Here's how the part is built. I have some questions about the finished solid (model axes, mm). A direction names the side the tool comes from. Coordinates: 2 decimals unless noted, no trailing zeros. Loops run counter-clockwise (first coordinate to the right, second up) from the corner with the lowest first, then second, coordinate; pieces in that order, holes last.
```python
from build123d import *

# Parameters (mm, degrees)
BOSS_EXTRUDE1_DEPTH = 12
CUT_EXTRUDE1_DEPTH  = 2
SKETCH3_W           = 16.6
SKETCH3_H           = 13.4
BOSS_EXTRUDE2_DEPTH = 5.2
SKETCH5_R           = 1.6
CUT_EXTRUDE2_DEPTH  = 5
SKETCH6_W           = 5
SKETCH6_H           = 4
BOSS_EXTRUDE4_DEPTH = 8
CUT_EXTRUDE4_DEPTH  = 7
SKETCH8_R           = 2.65
CUT_EXTRUDE5_DEPTH  = 7
SKETCH10_R          = 2.65
CUT_EXTRUDE6_DEPTH  = 7
CHAMFER2_SIZE       = 2
CHAMFER3_SIZE       = 1
SKETCH12_W          = 3
SKETCH12_H          = 2
SKETCH12_W_2        = 6.148694825
SKETCH12_W_3        = 1.851305175
BOSS_EXTRUDE5_DEPTH = 8
SKETCH13_R          = 2.65
CUT_EXTRUDE7_DEPTH  = 3
CHAMFER4_SIZE       = 5
CHAMFER4_SIZE_2     = 6.174485783
SKETCH16_W          = 1.5
SKETCH16_H          = 10
CUT_EXTRUDE8_DEPTH  = 11
CHAMFER5_SIZE       = 0.4


with BuildPart() as part:
    # Sketch1 → Boss-Extrude1 (new body)
    with BuildSketch(Plane(origin=(0, 0, 0), x_dir=(1, 0, 0), z_dir=(0, 1, 0))):
        with BuildLine():
            Line((-23.25, -5), (-5.749755012, -5))
            Line((-5.749755012, -5), (-5.749755012, 0))
            add(Edge.make_bspline(
                [(-3.25, 5), (-5.749755012, 5), (-5.749755012, 0)],
                knots=[0, 0, 0, 1.570796327, 1.570796327, 1.570796327], degree=2, weights=[1, 0.707106781, 1]))
            Line((-3.25, 5), (3.25, 5))
            add(Edge.make_bspline(
                [(5.748694825, 0), (5.748694825, 5), (3.25, 5)],
                knots=[4.71238898, 4.71238898, 4.71238898, 6.283185307, 6.283185307, 6.283185307], degree=2, weights=[1, 0.707106781, 1]))
            Line((5.748694825, 0), (5.748694825, -5))
            Line((5.748694825, -5), (23.25, -5))
            Line((23.25, -5), (23.25, -3))
            Line((23.25, -3), (23.25, -1))
            Line((23.25, -1), (9.3, -1))
            ThreePointArc((9.3, -1), (8.592893219, -0.707106781), (8.3, 0))
            Line((8.3, 0), (8.3, 6.6))
            Line((8.3, 6.6), (-8.3, 6.6))
            Line((-8.3, 6.6), (-8.3, 0))
            ThreePointArc((-8.3, 0), (-8.592893219, -0.707106781), (-9.3, -1))
            Line((-9.3, -1), (-23.25, -1))
            Line((-23.25, -1), (-23.25, -5))
        make_face()
    extrude(amount=BOSS_EXTRUDE1_DEPTH)

    # Sketch2 → Cut-Extrude1 (cut)
    with BuildSketch(Plane(origin=(0, 0, 1), x_dir=(-1, 0, 0), z_dir=(0, 0, -1))):
        Polygon((20.147177825, 6), (18.213054423, 9.35), (14.344807619, 9.35), (12.410684218, 6), (14.344807619, 2.65), (18.213054423, 2.65), align=None)
        Polygon((-12.542169585, 6), (-14.476292987, 9.35), (-18.34453979, 9.35), (-20.278663192, 6), (-18.34453979, 2.65), (-14.476292987, 2.65), align=None)
    extrude(amount=-CUT_EXTRUDE1_DEPTH, mode=Mode.SUBTRACT)

    # Sketch3 → Boss-Extrude2 (add)
    with BuildSketch(Plane(origin=(0, 12, 0), x_dir=(1, 0, 0), z_dir=(0, 1, 0))):
        with Locations((0, 13.3)):
            Rectangle(SKETCH3_W, SKETCH3_H)
    extrude(amount=-BOSS_EXTRUDE2_DEPTH)

    # Sketch5 → Cut-Extrude2 (cut)
    with BuildSketch(Plane(origin=(0, 0, 1), x_dir=(-1, 0, 0), z_dir=(0, 0, -1))):
        with Locations((-16.410416388, 6)):
            Circle(SKETCH5_R)
        with Locations((16.278931021, 6)):
            Circle(SKETCH5_R)
    extrude(amount=-CUT_EXTRUDE2_DEPTH, mode=Mode.SUBTRACT)

    # Sketch6 → Boss-Extrude4 (add)
    with BuildSketch(Plane(origin=(0, 12, 0), x_dir=(1, 0, 0), z_dir=(0, 1, 0))):
        with Locations((8.948694825, -3)):
            Rectangle(SKETCH6_W, SKETCH6_H)
    extrude(amount=BOSS_EXTRUDE4_DEPTH)

    # Sketch7 → Cut-Extrude4 (cut)
    with BuildSketch(Plane(origin=(0, 0, 1), x_dir=(-1, 0, 0), z_dir=(0, 0, -1))):
        with BuildLine():
            ThreePointArc((-6.448694825, 16), (-6.468205549, 16.252991544), (-6.526276305, 16.5))
            Line((-6.526276305, 16.5), (-7.999397269, 16.5))
            Line((-7.999397269, 16.5), (-7.999397269, 15.5))
            Line((-7.999397269, 15.5), (-6.526276305, 15.5))
            ThreePointArc((-6.526276305, 15.5), (-6.468205549, 15.747008456), (-6.448694825, 16))
        make_face()
        with BuildLine():
            Line((-7.999397269, 16.5), (-6.526276305, 16.5))
            ThreePointArc((-6.526276305, 16.5), (-9.748694825, 16), (-6.526276305, 15.5))
            Line((-6.526276305, 15.5), (-7.999397269, 15.5))
            Line((-7.999397269, 15.5), (-7.999397269, 16.5))
        make_face()
        with BuildLine():
            Line((-6.448694825, 15.5), (-6.448694825, 16))
            ThreePointArc((-6.448694825, 16), (-6.468205549, 15.747008456), (-6.526276305, 15.5))
            Line((-6.526276305, 15.5), (-6.448694825, 15.5))
        make_face()
        with BuildLine():
            Line((-6.448694825, 16), (-6.448694825, 16.5))
            Line((-6.448694825, 16.5), (-6.526276305, 16.5))
            ThreePointArc((-6.526276305, 16.5), (-6.468205549, 16.252991544), (-6.448694825, 16))
        make_face()
    extrude(amount=-CUT_EXTRUDE4_DEPTH, mode=Mode.SUBTRACT)

    # Sketch8 → Cut-Extrude5 (cut, along a direction that is not the sketch's normal)
    with BuildSketch(Plane(origin=(0, 12, 0), x_dir=(1, 0, 0), z_dir=(0, 1, 0))):
        with Locations((-4, 9.6)):
            Circle(SKETCH8_R)
    extrude(amount=-CUT_EXTRUDE5_DEPTH, dir=(0.2588190451025147, 0.96592582628907, -1.457918124587514e-13), mode=Mode.SUBTRACT)

    # Sketch10 → Cut-Extrude6 (cut, along a direction that is not the sketch's normal)
    with BuildSketch(Plane(origin=(0, 12, 0), x_dir=(1, 0, 0), z_dir=(0, 1, 0))):
        with Locations((4, 9.6)):
            Circle(SKETCH10_R)
    extrude(amount=-CUT_EXTRUDE6_DEPTH, dir=(-0.25881904510251447, 0.96592582628907, 0), mode=Mode.SUBTRACT)

    # Chamfer2
    chamfer2_edges = [part.edges().sort_by_distance(p)[0] for p in [
        (7.874347412, 12, 1),
    ]]
    chamfer(chamfer2_edges, length=CHAMFER2_SIZE)

    # Chamfer3
    chamfer3_edges = [part.edges().sort_by_distance(p)[0] for p in [
        (11.448694825, 16, 1),
    ]]
    chamfer(chamfer3_edges, length=CHAMFER3_SIZE)

    # Sketch12 → Boss-Extrude5 (add)
    with BuildSketch(Plane(origin=(0, 12, 0), x_dir=(1, 0, 0), z_dir=(0, 1, 0))):
        with Locations((4.948694825, 19)):
            Rectangle(SKETCH12_W, SKETCH12_H)
        with Locations((11.374347413, 19)):
            Rectangle(SKETCH12_W_2, SKETCH12_H)
        with Locations((7.374347413, 19)):
            Rectangle(SKETCH12_W_3, SKETCH12_H)
    extrude(amount=BOSS_EXTRUDE5_DEPTH)

    # Sketch13 → Cut-Extrude7 (cut)
    with BuildSketch(Plane(origin=(0, 0, -20), x_dir=(-1, 0, 0), z_dir=(0, 0, -1))):
        with Locations((-8.098694825, 16)):
            Circle(SKETCH13_R)
    extrude(amount=-CUT_EXTRUDE7_DEPTH, mode=Mode.SUBTRACT)

    # Chamfer4
    # the kernel refuses this chamfer: 6.174485783, 5 mm, written as the material it adds along each edge
    with BuildSketch(Plane(origin=(8.3, 12, -18), x_dir=(-0.037204697112204525, -0.9993076655929289, 0), z_dir=(0, 0, -1))) as chamfer4_piece_1_section:
        Polygon((CHAMFER4_SIZE * 0.999307665593, -CHAMFER4_SIZE * 0.0372046971122), (-CHAMFER4_SIZE_2 * 0.0372046971102, -CHAMFER4_SIZE_2 * 0.99930766554), (0, 0), align=None)
    chamfer4_piece_1 = extrude(amount=2, mode=Mode.PRIVATE)
    chamfer4_piece_1 = split(chamfer4_piece_1, bisect_by=Plane(origin=(14.448694825, 10.333304375, -19), z_dir=(-1, 0, 0)), keep=Keep.TOP, mode=Mode.PRIVATE)
    add(chamfer4_piece_1)

    # Sketch16 → Cut-Extrude8 (cut)
    with BuildSketch(Plane.XZ.offset(-6.8)):
        with Locations((0, -11.6)):
            Rectangle(SKETCH16_W, SKETCH16_H)
    extrude(amount=-CUT_EXTRUDE8_DEPTH, mode=Mode.SUBTRACT)

    # Chamfer5
    chamfer5_edges = [part.edges().sort_by_distance(p)[0] for p in [
        (0, 0, -5),
        (-5.260112096, 0, -2.972310439),
        (-5.749755012, 0, 2.5),
        (-14.499877506, 0, 5),
        (-23.25, 0, 3),
        (-16.275, 0, 1),
        (-8.592893219, 0, 0.707106781),
        (-8.3, 0, -3.3),
        (0, 0, -6.6),
        (8.3, 0, -3.3),
        (8.592893219, 0, 0.707106781),
        (16.275, 0, 1),
        (23.25, 0, 3),
        (14.499347412, 0, 5),
        (5.748694825, 0, 2.5),
        (5.259369228, 0, -2.972013605),
    ]]
    chamfer(chamfer5_edges, length=CHAMFER5_SIZE)


solid = part.part
```
1. I want a section at B-B (x = -19). Please give me the cut outline in (y, z).
2. I need wall thicknesses on line 1 along Z through (x, y) = (9.5, 12); line 2 along X through (y, z) = (7.5, -9.5); line 3 along X through (y, z) = (7.25, 3.5). Which ranges of each line are inside material? Lowest first, please.
3. On a 3-axis mill with a long thin cutter (end or side, diameter ignored), from which of +Z, -Z, +X, -X, +Y, -Y can I reach the whole of each face in a straight line? I mean faces 4 (the flat face through (16, 9.35, 2)), 5 (the flat face through (5.749, 6, 2)), 6 (the flat face through (10.94, 15.94, 1.49)). Say none if no direction works.
4. I want a section at C-C (y = 5.5). Give the number of separate pieces and of enclosed holes in the cut face, then the cut area to 3 significant figures.
5. For pin 1 (1.6 mm diameter, centred on x = -17, z = 2.5, fed in from +Y); pin 2 (3 mm diameter, centred on y = 10, z = -12, fed in from -X); pin 3 (5 mm diameter, centred on y = 11, z = -7, fed in from +X), each with a flat end and sliding along its axis, tell me the tip position at first contact or that it passes through.
6. I want a section at A-A (y = 16). Please give me the cut outline in (x, z), then the cut area to 3 significant figures.
7. We'd pull the mould along X, two halves only. Please class faces 1 (the cylindrical face through (8.601, 7.105, 0.715)), 2 (the flat face through (-16, 10, 1)), 3 (the flat face through (19.325, 4.348, 1.986)): +X half, -X half, draft (parallel to the pull), parting line (faces both ways), or undercut.
Response values:
1. outline: (0, 1.4) - (0.4, 1) - (4.01, 1) - (4.01, 3) - (7.99, 3) - (7.99, 1) - (12, 1) - (12, 5) - (0.4, 5) - (0, 4.6) - close
2. line 1: z = -20 to -18, 1 to 5
2. line 2: x = -8.3 to -7.85, -2.56 to -0.75, 0.75 to 2.56, 7.85 to 8.3
2. line 3: x = -23.25 to -17.28, -15.28 to -5.75, 5.75 to 15.41, 17.41 to 23.25
3. face 4: -Z
3. face 5: +Z, +Y, -Y
3. face 6: +X, +Y
4. separate pieces: 3
4. enclosed holes: 0
4. area: 162 mm2
5. pin 1: stops at y = 12
5. pin 2: stops at x = -8.3
5. pin 3: stops at x = 8.3
6. outline: (3.45, -20) - (5.45, -20) - (5.45, -18) - (3.45, -18) - close; (9.75, 1) - (10.45, 1) - (11.45, 2) - (11.45, 5) - (9.75, 5) - close; (10.75, -20) - (14.45, -20) - (14.45, -18) - (10.75, -18) - close
6. area: 17.7 mm2
7. face 1: +X half
7. face 2: draft
7. face 3: undercut
